The figure shows three views and two pictorial views of one solid part (mm, origin at its lowest corner). Answer the questions. Coordinates: 2 decimals unless noted, no trailing zeros. Order: outer loops, then holes, each group sorted by start corner. A loop starts at its lowest first (then second) coordinate and runs counter-clockwise, first axis right, second up. Notation, with made-up numbers: M 3.25,62.5 L 27.25,62.5 A28 ccw 27.25,99.5 Z; hole C 20,-38 d1. An arc over 180 degrees is marked long. Answer in a Markdown table with one row per item. Add a question column.
Item 1: The part is cut by section D-D (y = 4). Write down the section's boundary in (x, z) (1 decimal), then the cut area to 3 significant figures.
Item 2: The part is cut by section B-B (x = 25.25). State how many separate pieces and enclosed holes the cut face has, then the cut area to 3 significant figures.
Item 3: Consider line 1 (Y direction, x = 2.5, z = 4.25); line 2 (Z direction, x = 24.5, y = 14) (1 decimal); line 3 (X direction, y = 8.5, z = 3.75) (1 decimal). Determine where each line is inside the solid, lowest interval first. Write a range as from..to.
Item 4: The part is cut by section A-A (y = 9). Write down the section's boundary in (x, z) (1 decimal), then the cut area to 3 significant figures.
Item 5: The part is cut by section C-C (z = 2.5). Write down the section's boundary in (x, y) (1 decimal), then the cut area to 3 significant figures.
Item 6: Flat-ended cylindrical pins translate along their axes: pin 1 Ø1.8 at (y, z) = (3.5, 5) entering from +X (1 decimal); pin 2 Ø2 at (y, z) = (14, 4.76) entering from -X. Find the tip coordinate at first contact, or state that the pin passes through.
Item 7: The mould has two halves that part along X. Classify the marked faces 1, 2 and 3: released by +X, released by -X, zero draft, split by the parting line, or undercut.
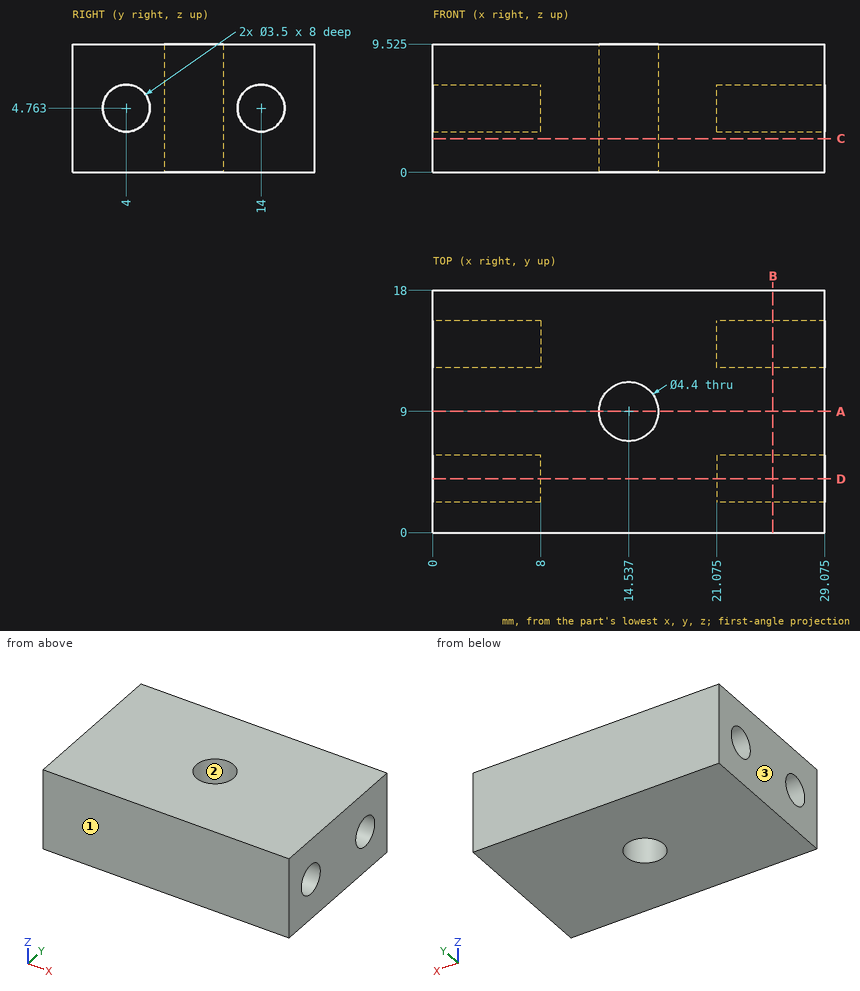
Reply:
| question | item | result |
|---|---|---|
| 1 | outline | M 0,0 L 29.1,0 L 29.1,3 L 21.1,3 L 21.1,6.5 L 29.1,6.5 L 29.1,9.5 L 0,9.5 L 0,6.5 L 8,6.5 L 8,3 L 0,3 Z |
| 1 | area | 221 mm2 |
| 2 | separate pieces | 1 |
| 2 | enclosed holes | 2 |
| 2 | area | 152 mm2 |
| 3 | line 1 | y = 0..2.33, 5.67..12.33, 15.67..18 |
| 3 | line 2 | z = 0..3, 6.5..9.5 |
| 3 | line 3 | x = 0..12.4, 16.7..29.1 |
| 4 | outline | M 0,0 L 12.3,0 L 12.3,9.5 L 0,9.5 Z; M 16.7,0 L 29.1,0 L 29.1,9.5 L 16.7,9.5 Z |
| 4 | area | 235 mm2 |
| 5 | outline | M 0,0 L 29.1,0 L 29.1,18 L 0,18 Z; hole C 14.5,9 d4.4 |
| 5 | area | 508 mm2 |
| 6 | pin 1 | stops at x = 21.1 |
| 6 | pin 2 | stops at x = 8 |
| 7 | face 1 | zero draft |
| 7 | face 2 | undercut |
| 7 | face 3 | released by -X |
